```python
from build123d import *

# Parameters (mm, degrees)
SKETCH_2_W               = 3.5
SKETCH_2_H               = 18
EXTRUDE_1_DEPTH          = 25
SKETCH_3_W               = 4.492765479
SKETCH_3_H               = 18
EXTRUDE_2_DEPTH          = 28
CUT_EXTRUDE_1_DEPTH      = 15
SKETCH_5_W               = 18
SKETCH_5_H               = 1.12
CUT_EXTRUDE_2_DEPTH      = 4
SKETCH_6_W               = 15.061219586
SKETCH_6_H               = 9.659551438
CUT_EXTRUDE_3_DEPTH      = 26
SKETCH_7_R               = 2.5
CUT_EXTRUDE_4_DEPTH      = 1
CUT_EXTRUDE_4_DEPTH_BACK = 32.5
SKETCH_8_W               = 15.061219586
SKETCH_8_H               = 1.746167636
CUT_EXTRUDE_5_DEPTH      = 5.566914265


with BuildPart() as part:
    # Эскиз2 → Бобышка-Вытянуть1 (new body)
    with BuildSketch(Plane.XY):
        with Locations((1.75, 9)):
            Rectangle(SKETCH_2_W, SKETCH_2_H)
    extrude(amount=EXTRUDE_1_DEPTH)

    # Эскиз3 → Бобышка-Вытянуть2 (add)
    with BuildSketch(Plane(origin=(3.5, 0, 0), x_dir=(0, 0, -1), z_dir=(1, 0, 0))):
        with Locations((-22.753617261, 9)):
            Rectangle(SKETCH_3_W, SKETCH_3_H)
    extrude(amount=EXTRUDE_2_DEPTH)

    # Эскиз4 → Вырез-Вытянуть1 (cut)
    with BuildSketch(Plane(origin=(0, 18, 0), x_dir=(1, 0, 0), z_dir=(0, 1, 0))):
        Polygon((4.95959575, -20.507234521), (4.95959575, -22.003832364), (3.55959575, -22.003832364), (3.55959575, -23.253832364), (28.98959575, -23.253832364), (28.98959575, -22.003832364), (27.48959575, -22.003832364), (27.48959575, -20.507234521), align=None)
    extrude(amount=-CUT_EXTRUDE_1_DEPTH, mode=Mode.SUBTRACT)

    # Эскиз5 → Вырез-Вытянуть2 (cut, through all)
    with BuildSketch(Plane(origin=(0, 3, 0), x_dir=(1, 0, 0), z_dir=(0, 1, 0))):
        with Locations((15.035669989, -22.124024477)):
            Rectangle(SKETCH_5_W, SKETCH_5_H)
    extrude(amount=-CUT_EXTRUDE_2_DEPTH, mode=Mode.SUBTRACT)

    # Эскиз6 → Вырез-Вытянуть3 (cut, through all)
    with BuildSketch(Plane.XY.offset(25)):
        with Locations((15.969390207, 8.603310016)):
            Rectangle(SKETCH_6_W, SKETCH_6_H)
    extrude(amount=-CUT_EXTRUDE_3_DEPTH, mode=Mode.SUBTRACT)

    # Эскиз7 → Вырез-Вытянуть4 (cut, two sides)
    with BuildSketch(Plane.ZY) as cut_extrude_4_sk:
        with Locations((5.030711772, 9)):
            Circle(SKETCH_7_R)
    extrude(amount=CUT_EXTRUDE_4_DEPTH, mode=Mode.SUBTRACT)
    extrude(cut_extrude_4_sk.sketch, amount=-CUT_EXTRUDE_4_DEPTH_BACK, mode=Mode.SUBTRACT)

    # Эскиз8 → Вырез-Вытянуть5 (cut, through all)
    with BuildSketch(Plane.XZ.offset(-13.433085735)):
        with Locations((15.969390207, 24.126916182)):
            Rectangle(SKETCH_8_W, SKETCH_8_H)
    extrude(amount=-CUT_EXTRUDE_5_DEPTH, mode=Mode.SUBTRACT)


solid = part.part
```
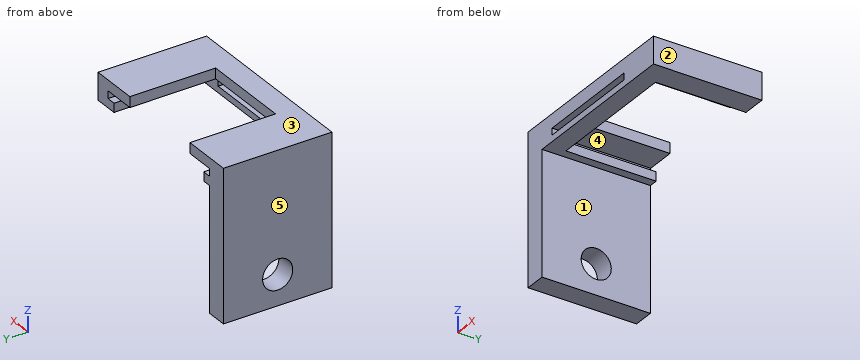
For this review, take the finished solid that the model builds, in its own axes (mm). Face numbers are marked on the shaded views. A direction names the side the tool comes from. Give positions to 0.01 mm unless a question says otherwise; leave off trailing zeros. Order: outer loops, then holes, each group sorted by start corner. A loop starts at its lowest first (then second) coordinate and runs counter-clockwise, first axis right, second up.
1) Take a section at A-A (y = 1.75). Give the boundary of the cut face in (x, z).
2) Take a section at D-D (z = 6). Give the boundary of the cut face in (x, y).
3) Wall thickness on line 1 (Z direction, x = 28.5, y = 12.25); line 2 (Z direction, x = 11.5, y = 1.5); line 3 (X direction, y = 5, z = 8): over which ranges is each line inside the solid? List them lowest first.
4) Insertion check: pin 1 (6 mm diameter, centred on x = 12.5, y = 11.5, fed in from +Z); pin 2 (0.9 mm diameter, centred on y = 10.5, z = 24, fed in from -X); pin 3 (2 mm diameter, centred on x = 16, z = 22.5, fed in from +Y); pin 4 (1.5 mm diameter, centred on x = 11.5, y = 1.5, fed in from -Z). Each pin has a flat end and moves straight along its axis. Give the tip position at first contact, or say it passes through.
5) Take a section at B-B (x = 10.5). Give the boundary of the cut face in (y, z).
6) For the marked faces 1 and 2, list the 3-axis set-ups (+Z, -Z, +X, -X, +Y, -Y) from which the entire face can be reached by the end or side of a thin tool; tool diameter is ignored.
7) The part is to be moulded in two halves that separate along Z. For the marked faces 3, 4 and 5, say which applies: released by +Z, released by -Z, zero draft, split by the parting line, or undercut.
8) Take a section at C-C (y = 9). Give the boundary of the cut face in (x, z), then the cut area to 3 significant figures.
Derived:
1. outline: (0, 0) - (3.5, 0) - (3.5, 20.51) - (31.5, 20.51) - (31.5, 25) - (0, 25) - close; hole (6.04, 21.56) - (24.04, 21.56) - (24.04, 22.68) - (6.04, 22.68) - close
2. outline: (0, 0) - (3.5, 0) - (3.5, 6.7) - (0, 6.7) - close; (0, 11.3) - (3.5, 11.3) - (3.5, 18) - (0, 18) - close
3. line 1: z = 20.51 to 22, 23.25 to 25
3. line 2: z = 20.51 to 21.56, 22.68 to 25
3. line 3: x = 0 to 3.5
4. pin 1: passes through
4. pin 2: stops at x = 0
4. pin 3: stops at y = 3.77
4. pin 4: stops at z = 20.51
5. outline: (0, 20.51) - (3, 20.51) - (3, 21.56) - (0, 21.56) - close; (0, 22.68) - (3, 22.68) - (3, 23.25) - (3.77, 23.25) - (3.77, 25) - (0, 25) - close
6. face 1: -Z, +X, +Y, -Y
6. face 2: +Z, -Z, +X, +Y, -Y
7. face 3: released by +Z
7. face 4: undercut
7. face 5: zero draft
8. outline: (0, 0) - (3.5, 0) - (3.5, 2.53) - (0, 2.53) - close; (0, 7.53) - (3.5, 7.53) - (3.5, 20.51) - (4.96, 20.51) - (4.96, 22) - (3.56, 22) - (3.56, 23.25) - (8.44, 23.25) - (8.44, 25) - (0, 25) - close; (23.5, 23.25) - (28.99, 23.25) - (28.99, 22) - (27.49, 22) - (27.49, 20.51) - (31.5, 20.51) - (31.5, 25) - (23.5, 25) - close
8. area: 104 mm2
